Part model, mm, in its own coordinate system. A direction names the side the tool comes from. Give positions to 0.01 mm unless a question says otherwise; leave off trailing zeros. Write each loop counter-clockwise with the first axis right and the second up, starting at its lowest first coordinate (ties: lowest second). Pieces come first, ordered by that corner, then holes. Notation, with made-up numbers: M -19,-27.75 L 18,-27.75 A29 cw 18,5.25 Z; hole C 7.25,-18.75 d4. An arc over 180 degrees is marked long. Use CSV: the item, a comma, the result in double quotes. Start each with the question number.
Item 1: Drill centre lines: line 1 (X direction, y = -65, z = 0.8); line 2 (X direction, y = -21, z = 1.85); line 3 (Y direction, x = -68, z = 1.05). Where is each one in solid material? Low to high. Write a range as [from, to].
Item 2: Mould opens along X. For faces 1 (the flat face through (-18, -14, 0)), 2 (the flat face through (-58, -80, 2)), 3 (the flat face through (78, -65, 2)), 4 (the cylindrical face through (65.6, -21.8, 1)) say: released by +X, released by -X, zero draft, split by the parting line, or undercut.
Item 3: Cut at B-B (z = 2.65). Count the separate pieces of the cut face and the enclosed holes in it, then the cut area to 3 significant figures.
Item 4: Pin check, flat tips, straight feed: pin 1 (5.5 mm diameter, centred on x = 68, y = -20, fed in from -Z); pin 2 (1.2 mm diameter, centred on y = -7, z = 2.5, fed in from +X); pin 3 (9.5 mm diameter, centred on x = -68, y = -20, fed in from -Z); pin 4 (0.8 mm diameter, centred on x = 17.5, z = 2, fed in from -Y). Stop position of each tip, or through.
Item 5: Cut at A-A (y = -100). List the corners of the cut face in (x, z).
Item 6: Which spindle directions (+Z, -Z, +X, -X, +Y, -Y) get a long thin tool onto all of the face, cutting with end or side? Do faces 5 (the flat face through (38.15, -37.32, 1.97)), 6 (the flat face through (-57.5, -7, 2)), 7 (the flat face through (68, -10, 2)), 8 (the conical face through (-65.019, -19.061, 2.125)). Say none if no direction does.
Item 7: Cut at C-C (x = 68). List the corners of the cut face in (y, z).
Item 8: Cut at D-D (y = -64). List the corners of the cut face in (x, z), then the cut area to 3 significant figures.
from build123d import *

# Parameters (mm, degrees)
SKETCH_R     = 3
PAD_DEPTH    = 4
CHAMFER_SIZE = 2


with BuildPart() as part:
    # Sketch → Pad (new body)
    with BuildSketch(Plane.XY):
        with BuildLine():
            Line((-78, -10), (-78, -119.313708))
            ThreePointArc((-78, -119.313708), (-76.765367, -121.161468), (-74.585786, -120.727922))
            Line((-74.585786, -120.727922), (-58.585786, -104.727922))
            ThreePointArc((-58.585786, -104.727922), (-58.152241, -104.079075), (-58, -103.313708))
            Line((-58, -58), (-58, -103.313708))
            ThreePointArc((-57.414214, -56.585786), (-57.847759, -57.234633), (-58, -58))
            Line((-57.414214, -56.585786), (-19.414214, -18.585786))
            ThreePointArc((-18, -18), (-18.765367, -18.152241), (-19.414214, -18.585786))
            Line((-18, -18), (-17, -18))
            ThreePointArc((-17, -18), (-15.585786, -17.414214), (-15, -16))
            Line((-15, -16), (-15, -12))
            ThreePointArc((-13, -10), (-14.414214, -10.585786), (-15, -12))
            Line((-13, -10), (13, -10))
            ThreePointArc((15, -12), (14.414214, -10.585786), (13, -10))
            Line((15, -16), (15, -12))
            ThreePointArc((15, -16), (15.585786, -17.414214), (17, -18))
            Line((17, -18), (18, -18))
            ThreePointArc((19.414214, -18.585786), (18.765367, -18.152241), (18, -18))
            Line((19.414214, -18.585786), (57.414214, -56.585786))
            ThreePointArc((58, -58), (57.847759, -57.234633), (57.414214, -56.585786))
            Line((58, -58), (58, -103.313708))
            ThreePointArc((58, -103.313708), (58.152241, -104.079075), (58.585786, -104.727922))
            Line((58.585786, -104.727922), (74.585786, -120.727922))
            ThreePointArc((74.585786, -120.727922), (76.765367, -121.161468), (78, -119.313708))
            Line((78, -119.313708), (78, -10))
            Line((57.5, -10), (78, -10))
            Line((57.5, -3), (57.5, -10))
            Line((57.5, -3), (-57.5, -3))
            Line((-57.5, -10), (-57.5, -3))
            Line((-78, -10), (-57.5, -10))
        make_face()
        with Locations((-68, -20)):
            Circle(SKETCH_R, mode=Mode.SUBTRACT)
        with Locations((-68, -100)):
            Circle(SKETCH_R, mode=Mode.SUBTRACT)
        with Locations((68, -20)):
            Circle(SKETCH_R, mode=Mode.SUBTRACT)
        with Locations((68, -100)):
            Circle(SKETCH_R, mode=Mode.SUBTRACT)
    extrude(amount=PAD_DEPTH)

    # Chamfer
    chamfer_edges = [part.edges().sort_by_distance(p)[0] for p in [
        (-71, -20, 4),
        (65, -20, 4),
    ]]
    chamfer(chamfer_edges, length=CHAMFER_SIZE)


solid = part.part
Worked answers:
1,line 1,"x = [-78, -58], [58, 78]"
1,line 2,"x = [-78, -70.83], [-65.17, -21.83], [21.83, 65.17], [70.83, 78]"
1,line 3,"y = [-114.14, -103], [-97, -23], [-17, -10]"
2,face 1,"zero draft"
2,face 2,"undercut"
2,face 3,"released by +X"
2,face 4,"undercut"
3,separate pieces,"1"
3,enclosed holes,"4"
3,area,"7,040 mm^2"
4,pin 1,"passes through"
4,pin 2,"stops at x = 57.5"
4,pin 3,"stops at z = 0"
4,pin 4,"stops at y = -18"
5,outline,"M -78,0 L -71,0 L -71,4 L -78,4 Z; M -65,0 L -58,0 L -58,4 L -65,4 Z; M 58,0 L 65,0 L 65,4 L 58,4 Z; M 71,0 L 78,0 L 78,4 L 71,4 Z"
6,face 5,"+Z, -Z, -Y"
6,face 6,"+Z, -Z, -X, +Y"
6,face 7,"+Z, -Z, +X, +Y"
6,face 8,"+Z"
7,outline,"M -114.14,0 L -103,0 L -103,4 L -114.14,4 Z; M -97,0 L -23,0 L -23,2 L -25,4 L -97,4 Z; M -17,0 L -10,0 L -10,4 L -15,4 L -17,2 Z"
8,outline,"M -78,0 L -58,0 L -58,4 L -78,4 Z; M 58,0 L 78,0 L 78,4 L 58,4 Z"
8,area,"160 mm^2"
